from build123d import *

# Parameters (mm, degrees)
EXTRUDE_1_DEPTH     = 10
CUT_EXTRUDE_1_DEPTH = 8.5
SKETCH_3_R          = 2.2
CUT_EXTRUDE_2_DEPTH = 11


with BuildPart() as part:
    # Эскиз1 → Бобышка-Вытянуть1 (new body)
    with BuildSketch(Plane(origin=(0, 0, 0), x_dir=(1, 0, 0), z_dir=(0, 1, 0))):
        with BuildLine():
            Line((-40, 43), (40, 43))
            ThreePointArc((40, 43), (42.121320344, 42.121320344), (43, 40))
            Line((43, 40), (43, -40))
            ThreePointArc((43, -40), (42.121320344, -42.121320344), (40, -43))
            Line((40, -43), (-40, -43))
            ThreePointArc((-40, -43), (-42.121320344, -42.121320344), (-43, -40))
            Line((-43, -40), (-43, 40))
            ThreePointArc((-43, 40), (-42.121320344, 42.121320344), (-40, 43))
        make_face()
    extrude(amount=EXTRUDE_1_DEPTH)

    # Эскиз2 → Вырез-Вытянуть1 (cut)
    with BuildSketch(Plane(origin=(0, 10, 0), x_dir=(1, 0, 0), z_dir=(0, 1, 0))):
        with BuildLine():
            Line((-38.5, -41.5), (38.5, -41.5))
            ThreePointArc((38.5, -41.5), (40.621320344, -40.621320344), (41.5, -38.5))
            Line((41.5, -38.5), (41.5, 38.5))
            ThreePointArc((41.5, 38.5), (40.621320344, 40.621320344), (38.5, 41.5))
            Line((38.5, 41.5), (-38.5, 41.5))
            ThreePointArc((-38.5, 41.5), (-40.621320344, 40.621320344), (-41.5, 38.5))
            Line((-41.5, 38.5), (-41.5, -38.5))
            ThreePointArc((-41.5, -38.5), (-40.621320344, -40.621320344), (-38.5, -41.5))
        make_face()
    extrude(amount=-CUT_EXTRUDE_1_DEPTH, mode=Mode.SUBTRACT)

    # Эскиз3 → Вырез-Вытянуть2 (cut, through all)
    with BuildSketch(Plane.XZ):
        with Locations((-15, 20)):
            Circle(SKETCH_3_R)
        with Locations((15, 20)):
            Circle(SKETCH_3_R)
    extrude(amount=-CUT_EXTRUDE_2_DEPTH, mode=Mode.SUBTRACT)


solid = part.part
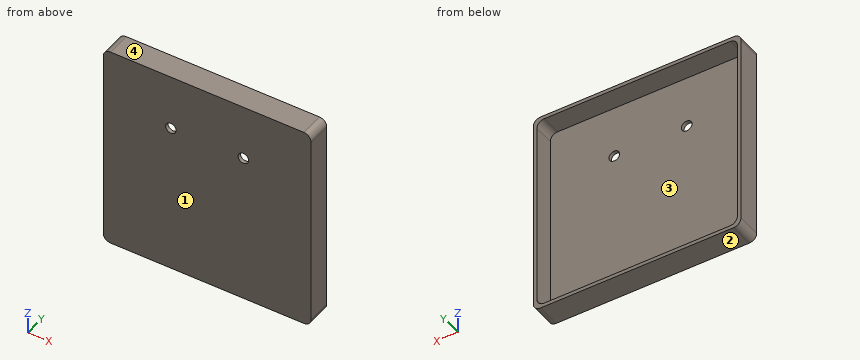
Here's how the part is built. I have some questions about the finished solid (model axes, mm). Face numbers are marked on the shaded views. Give positions to 0.01 mm unless a question says otherwise; leave off trailing zeros. Order: outer loops, then holes, each group sorted by start corner. A loop starts at its lowest first (then second) coordinate and runs counter-clockwise, first axis right, second up. Notation, with made-up numbers: (-14.75, -34.5) -> (31.25, -34.5) arc R23 cw to (31.25, 3.5) -> close; hole circle Ø1 at (44, 37.5). An arc over 180 degrees is marked (long way). One line per item, written item: value. Start each with the question number.
1. Imagine slicing it at C-C, the plane y = 6. List the corners of the cut face in (x, z) for me, plus the area to 3 significant figures.
2. Imagine slicing it at D-D, the plane x = -36. List the corners of the cut face in (y, z) for me, plus the area to 4 significant figures.
3. We'd pull the mould along Z, two halves only. Please class the marked faces 1, 2, 3 and 4: released by +Z, released by -Z, zero draft, split by the parting line, or undercut.
4. Imagine slicing it at A-A, the plane z = 20. List the corners of the cut face in (x, y) for me, plus the area to 3 significant figures.
5. Imagine slicing it at B-B, the plane x = 15. List the corners of the cut face in (y, z) for me, plus the area to 3 significant figures.
6. Will these pins go through, and if not, where does the flat tip stop? pin 1 Ø6 at (x, z) = (-2.5, -30) entering from -Y; pin 2 Ø3.5 at (x, z) = (15, 20) entering from +Y (3 decimals); pin 3 Ø25 at (x, z) = (0.5, -6.5) entering from +Y.
7. I need wall thicknesses on probe 1 along Z at (x, y) = (-26, 9); probe 2 along Z at (x, y) = (15, 0.4). Which ranges of each line are inside material? Lowest first, please. Write a range as from..to.
Values follow:
1. outline: (-43, -40) arc R3 ccw to (-40, -43) -> (40, -43) arc R3 ccw to (43, -40) -> (43, 40) arc R3 ccw to (40, 43) -> (-40, 43) arc R3 ccw to (-43, 40) -> close; hole (-41.5, -38.5) arc R3 ccw to (-38.5, -41.5) -> (38.5, -41.5) arc R3 ccw to (41.5, -38.5) -> (41.5, 38.5) arc R3 ccw to (38.5, 41.5) -> (-38.5, 41.5) arc R3 ccw to (-41.5, 38.5) -> close
1. area: 507 mm2
2. outline: (0, -43) -> (10, -43) -> (10, -41.5) -> (1.5, -41.5) -> (1.5, 41.5) -> (10, 41.5) -> (10, 43) -> (0, 43) -> close
2. area: 154.5 mm2
3. face 1: zero draft
3. face 2: released by -Z
3. face 3: undercut
3. face 4: released by +Z
4. outline: (-43, 0) -> (-17.2, 0) -> (-17.2, 1.5) -> (-41.5, 1.5) -> (-41.5, 10) -> (-43, 10) -> close; (-12.8, 0) -> (12.8, 0) -> (12.8, 1.5) -> (-12.8, 1.5) -> close; (17.2, 0) -> (43, 0) -> (43, 10) -> (41.5, 10) -> (41.5, 1.5) -> (17.2, 1.5) -> close
4. area: 141 mm2
5. outline: (0, -43) -> (10, -43) -> (10, -41.5) -> (1.5, -41.5) -> (1.5, 17.8) -> (0, 17.8) -> close; (0, 22.2) -> (1.5, 22.2) -> (1.5, 41.5) -> (10, 41.5) -> (10, 43) -> (0, 43) -> close
5. area: 148 mm2
6. pin 1: stops at y = 0
6. pin 2: passes through
6. pin 3: stops at y = 1.5
7. probe 1: z = -43..-41.5, 41.5..43
7. probe 2: z = -43..17.8, 22.2..43
